```python
from build123d import *

# Parameters (mm, degrees)
EXTRUSION1_DEPTH = 40.6


with BuildPart() as part:
    # Esquisse1 → Extrusion1 (new, symmetric)
    with BuildSketch(Plane.XY):
        with BuildLine():
            Line((-47.575077806, -19.430156076), (-47.575077806, 85.569843924))
            ThreePointArc((-47.575077806, 85.569843924), (-46.110611712, 89.10537783), (-42.575077806, 90.569843924))
            Line((-42.575077806, 90.569843924), (33.924922194, 90.569843924))
            Line((33.924922194, 90.569843924), (33.924922194, 87.569843924))
            Line((33.924922194, 87.569843924), (-42.575077806, 87.569843924))
            ThreePointArc((-42.575077806, 87.569843924), (-43.989291368, 86.984057487), (-44.575077806, 85.569843924))
            Line((-44.575077806, 85.569843924), (-44.575077806, -19.430156076))
            ThreePointArc((-44.575077806, -19.430156076), (-43.989291368, -20.844369638), (-42.575077806, -21.430156076))
            Line((-42.575077806, -21.430156076), (33.924922194, -21.430156076))
            Line((33.924922194, -21.430156076), (33.924922194, -24.430156076))
            Line((33.924922194, -24.430156076), (-42.575077806, -24.430156076))
            ThreePointArc((-42.575077806, -24.430156076), (-46.110611712, -22.965689982), (-47.575077806, -19.430156076))
        make_face()
    extrude(amount=EXTRUSION1_DEPTH, both=True)


solid = part.part
```
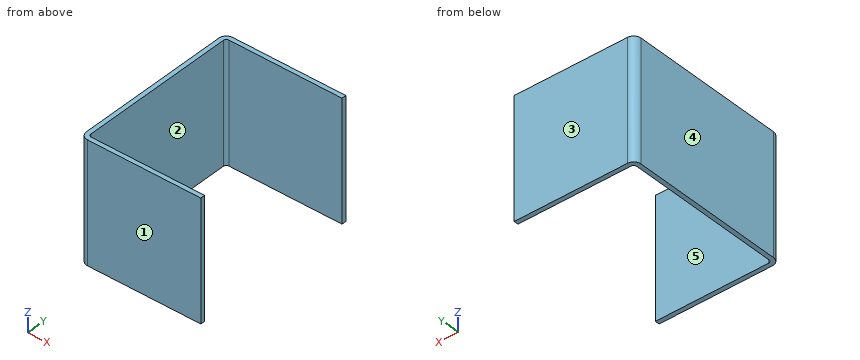
CAD build for the part. Positions are in the model's coordinates, mm. Face numbers are marked on the shaded views. A direction names the side the tool comes from. Round coordinates to 2 decimals unless told otherwise and drop trailing zeros. Loops run counter-clockwise (first coordinate to the right, second up) from the corner with the lowest first, then second, coordinate; pieces in that order, holes last. Notation, with made-up numbers: M 64,19 L 70,19 A37 cw 70,56 Z; hole C -10.75,42.5 d4. An arc over 180 degrees is marked long. Return JSON: item names as keys, results as strings. Group by question number.
(1) Tool access for the marked faces 1 and 2: list every direction of +Z, -Z, +X, -X, +Y, -Y with a clear straight run to the whole face (end or side of a thin tool).
(2) Saw through at B-B, the plane z = -31.5. List the corners of the cut face in (x, y), and give its area (3 significant figures).
(3) Saw through at C-C, the plane y = 78.5. List the corners of the cut face in (x, z), and give its area (3 significant figures).
(4) Wall check: probe 1 along Y at (x, z) = (6, -12.5); probe 2 along X at (y, z) = (0, 20.5). Give the ranges that are in metal, low to high. Write a range as [from, to].
(5) Mould opens along Y. For the marked faces 3, 4 and 5 say: +Y half, -Y half, draft (parallel to the pull), parting line (faces both ways), or undercut.
(6) Saw through at A-A, the plane x = -29.5. List the corners of the cut face in (y, z).
Answer list:
{
 "1": {"face 1": "+Z, -Z, +X, -X, -Y", "face 2": "+Z, -Z, +X"},
 "2": {"outline": "M -47.58,-19.43 A5 ccw -42.58,-24.43 L 33.92,-24.43 L 33.92,-21.43 L -42.58,-21.43 A2 cw -44.58,-19.43 L -44.58,85.57 A2 cw -42.58,87.57 L 33.92,87.57 L 33.92,90.57 L -42.58,90.57 A5 ccw -47.58,85.57 Z", "area": "807 mm2"},
 "3": {"outline": "M -47.58,-40.6 L -44.58,-40.6 L -44.58,40.6 L -47.58,40.6 Z", "area": "244 mm2"},
 "4": {"probe 1": "[-24.43, -21.43], [87.57, 90.57]", "probe 2": "[-47.58, -44.58]"},
 "5": {"face 3": "+Y half", "face 4": "draft", "face 5": "undercut"},
 "6": {"outline": "M -24.43,-40.6 L -21.43,-40.6 L -21.43,40.6 L -24.43,40.6 Z; M 87.57,-40.6 L 90.57,-40.6 L 90.57,40.6 L 87.57,40.6 Z"}
}
